The model under review builds one solid part; all positions refer to its coordinate system, in mm. A direction names the side the tool comes from. Round coordinates to 2 decimals unless told otherwise and drop trailing zeros. Order: outer loops, then holes, each group sorted by start corner. A loop starts at its lowest first (then second) coordinate and runs counter-clockwise, first axis right, second up. Notation, with made-up numbers: M -22,-2.5 L 9,-2.5 A5 ccw 9,2.5 Z; hole C 43.5,51.25 d9. An arc over 180 degrees is marked long. Answer as a JSON object with one key per item and string values. Group by question number.
1) Consider section B-B, the plane x = -1. Write out the cut boundary in (y, z), then the cut area to 3 significant figures.
2) Consider section D-D, the plane z = -4.25. Write out the cut boundary in (x, y).
3) To check wall thickness, follow line 1 (X direction, y = 10, z = -1.75); line 2 (Y direction, x = -4.75, z = 2); line 3 (Z direction, x = -10, y = 3). State the ranges of each line that lie inside material, in increasing order.
4) For faces 5 (the flat face through (-11, 9, 0)), 6 (the flat face through (-3, 12.35, 3)), 7 (the flat face through (-5.5, 9, 3)), 8 (the flat face through (-12, 4, 1.7)), list the 3-axis set-ups (+Z, -Z, +X, -X, +Y, -Y) from which the entire face can be reached by the end or side of a thin tool; tool diameter is ignored.
5) The part is to be moulded in two halves that separate along X. For faces 1 (the flat face through (1.5, 9, 3)), 2 (the flat face through (1, 9, 1.2)), 3 (the flat face through (-20.6, 9, -1)), 4 (the flat face through (-18.1, 9, -1)), say which applies: +X half, -X half, draft (parallel to the pull), parting line (faces both ways), or undercut.
6) Consider section C-C, the plane y = 5.25. Write out the cut boundary in (x, z), then the cut area to 3 significant figures.
7) Insertion check: pin 1 Ø1 at (x, y) = (-14.5, 8.5) entering from +Z; pin 2 Ø1.5 at (x, y) = (-21, 12.5) entering from -Z; pin 3 Ø4 at (x, y) = (-11, 15.5) entering from -Z. Each pin has a flat end and moves straight along its axis. Give the tip position at first contact, or say it passes through.
8) Consider section A-A, the plane z = -2. Write out the cut boundary in (x, y), then the cut area to 3 significant figures.
```python
from build123d import *

# Parameters (mm, degrees)
ESQUISSE1_W             = 22
ESQUISSE1_H             = 17.3
BOSS_EXTRU_1_DEPTH      = 1.2
ESQUISSE2_W             = 5.5
ESQUISSE2_H             = 7.4
ESQUISSE2_W_2           = 1.5
BOSS_EXTRU_2_DEPTH      = 2.73
ESQUISSE5_W             = 2
ESQUISSE5_H             = 4
ESQUISSE5_W_2           = 0.5
ESQUISSE5_H_2           = 1.5
ESQUISSE5_W_3           = 5
ESQUISSE5_H_3           = 3
ESQUISSE5_W_4           = 1.5
ESQUISSE5_H_4           = 0.5
ESQUISSE5_W_5           = 0.43407564
ESQUISSE5_H_5           = 1.061073785
ESQUISSE5_W_6           = 3.5
ESQUISSE5_H_6           = 5
BOSS_EXTRU_5_DEPTH      = 0.5
ENL_V_MAT_EXTRU_4_DEPTH = 2
ESQUISSE11_W            = 2.5
ESQUISSE11_H            = 17.3
BOSS_EXTRU_8_DEPTH      = 2.5
ESQUISSE12_R            = 0.25
BOSS_EXTRU_9_DEPTH      = 5


with BuildPart() as part:
    # Esquisse1 → Boss.-Extru.1 (new body)
    with BuildSketch(Plane.XY):
        with Locations((-11, 8.65)):
            Rectangle(ESQUISSE1_W, ESQUISSE1_H)
    extrude(amount=BOSS_EXTRU_1_DEPTH)

    # Esquisse2 → Boss.-Extru.2 (add)
    with BuildSketch(Plane.XY.offset(1.2)):
        with Locations((-2.75, 8.65)):
            Rectangle(ESQUISSE2_W, ESQUISSE2_H)
        with Locations((0.75, 8.65)):
            Rectangle(ESQUISSE2_W_2, ESQUISSE2_H)
    extrude(amount=BOSS_EXTRU_2_DEPTH)

    # Esquisse5 → Boss.-Extru.5 (add)
    with BuildSketch(Plane.XY.offset(1.2)):
        with Locations((-11.5, 4)):
            Rectangle(ESQUISSE5_W, ESQUISSE5_H)
        with Locations((-15.75, 1.25)):
            Rectangle(ESQUISSE5_W_2, ESQUISSE5_H_2)
        with Locations((-16.75, 1.25)):
            Rectangle(ESQUISSE5_W_2, ESQUISSE5_H_2)
        with Locations((-15.75, 3.25)):
            Rectangle(ESQUISSE5_W_2, ESQUISSE5_H_2)
        with Locations((-16.75, 3.25)):
            Rectangle(ESQUISSE5_W_2, ESQUISSE5_H_2)
        with Locations((-14.5, 13.8)):
            Rectangle(ESQUISSE5_W_3, ESQUISSE5_H_3)
        with Locations((-10.75, 15.55)):
            Rectangle(ESQUISSE5_W_4, ESQUISSE5_H_4)
        with Locations((-19.944355947, 11.67647182)):
            Rectangle(ESQUISSE5_W_5, ESQUISSE5_H_5)
        with Locations((-8.75, 9.3)):
            Rectangle(ESQUISSE5_W_6, ESQUISSE5_H_6)
    extrude(amount=BOSS_EXTRU_5_DEPTH)

    # Esquisse8 → Enlèv. mat.-Extru.4 (cut)
    with BuildSketch(Plane(origin=(1.5, 0, 0), x_dir=(0, 0, -1), z_dir=(1, 0, 0))):
        Polygon((-1.2, 6.45), (-1.2, 4.95), (-1.7, 4.95), align=None)
        Polygon((-1.2, 10.85), (-1.7, 12.35), (-1.2, 12.35), align=None)
        Polygon((-3.93, 4.95), (-3.93, 5.95), (-3.43, 4.95), align=None)
        Polygon((-3.93, 11.35), (-3.43, 12.35), (-3.93, 12.35), align=None)
    extrude(amount=-ENL_V_MAT_EXTRU_4_DEPTH, mode=Mode.SUBTRACT)

    # Esquisse11 → Boss.-Extru.8 (add)
    with BuildSketch(Plane(origin=(0, 0, 0), x_dir=(-1, 0, 0), z_dir=(0, 0, -1))):
        with Locations((1.85, 8.65)):
            Rectangle(ESQUISSE11_W, ESQUISSE11_H)
        with Locations((19.35, 8.65)):
            Rectangle(ESQUISSE11_W, ESQUISSE11_H)
    extrude(amount=BOSS_EXTRU_8_DEPTH)

    # Esquisse12 → Boss.-Extru.9 (add)
    with BuildSketch(Plane(origin=(0, 0, -2.5), x_dir=(-1, 0, 0), z_dir=(0, 0, -1))):
        with Locations(Location((1.85, 2.4, 0), (0, 0, 180))):
            Circle(ESQUISSE12_R)
        with Locations(Location((1.85, 14.9, 0), (0, 0, 180))):
            Circle(ESQUISSE12_R)
        with Locations(Location((19.35, 14.9, 0), (0, 0, 180))):
            Circle(ESQUISSE12_R)
        with Locations(Location((19.35, 2.4, 0), (0, 0, 180))):
            Circle(ESQUISSE12_R)
    extrude(amount=BOSS_EXTRU_9_DEPTH)


solid = part.part
```
Results list:
{
 "1": {"outline": "M 0,-2.5 L 17.3,-2.5 L 17.3,1.2 L 12.35,1.2 L 12.35,3.93 L 4.95,3.93 L 4.95,1.2 L 0,1.2 Z", "area": "84.2 mm^2"},
 "2": {"outline": "C -19.35,2.4 d0.5; C -19.35,14.9 d0.5; C -1.85,2.4 d0.5; C -1.85,14.9 d0.5"},
 "3": {"line 1": "-20.6 to -18.1, -3.1 to -0.6", "line 2": "4.95 to 12.35", "line 3": "0 to 1.2"},
 "4": {"face 5": "-Z, +Y, -Y", "face 6": "+Z, +X, +Y", "face 7": "+Z, +Y, -Y", "face 8": "+Z, -X, +Y, -Y"},
 "5": {"face 1": "+X half", "face 2": "draft", "face 3": "-X half", "face 4": "undercut"},
 "6": {"outline": "M -22,0 L -20.6,0 L -20.6,-2.5 L -18.1,-2.5 L -18.1,0 L -3.1,0 L -3.1,-2.5 L -0.6,-2.5 L -0.6,0 L 0,0 L 0,1.2 L -0.5,1.2 L -0.5,1.6 L 1.5,1.6 L 1.5,3.58 L -0.5,3.58 L -0.5,3.93 L -5.5,3.93 L -5.5,1.2 L -10.5,1.2 L -10.5,1.7 L -12.5,1.7 L -12.5,1.2 L -22,1.2 Z", "area": "57.5 mm^2"},
 "7": {"pin 1": "z = 1.2", "pin 2": "z = -2.5", "pin 3": "z = 0"},
 "8": {"outline": "M -20.6,0 L -18.1,0 L -18.1,17.3 L -20.6,17.3 Z; M -3.1,0 L -0.6,0 L -0.6,17.3 L -3.1,17.3 Z", "area": "86.5 mm^2"}
}
